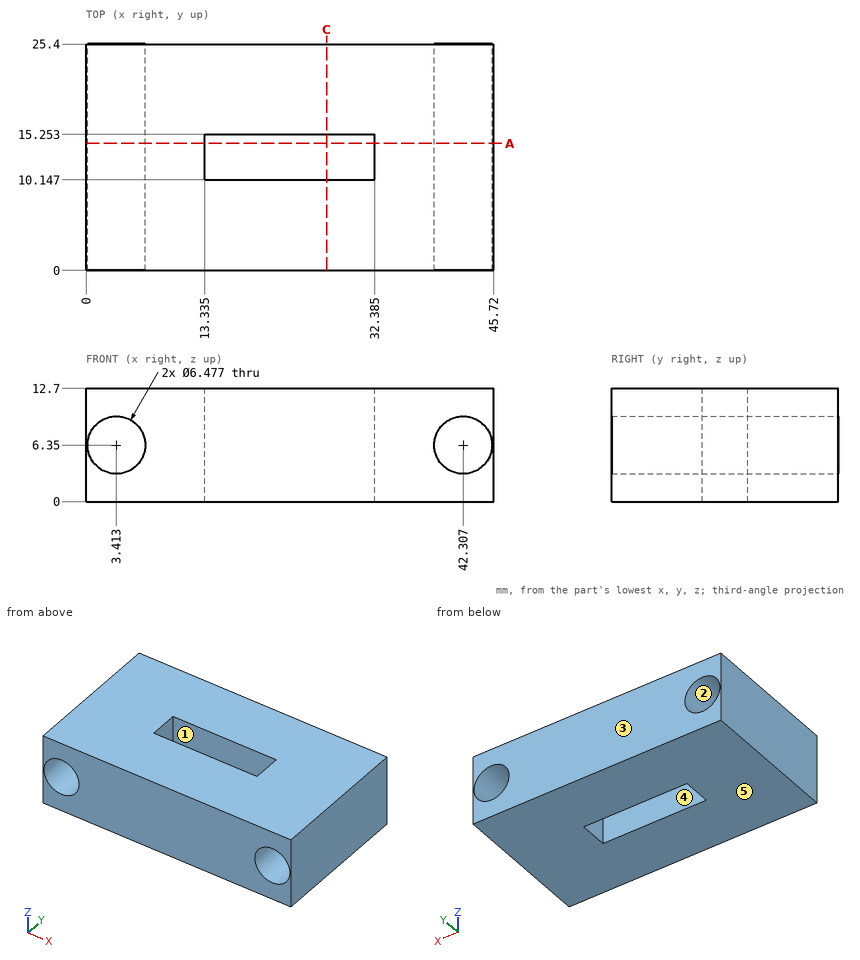
Source: three-view drawing plus pictorial views. Frame: mm from the lowest corner of the part. A direction names the side the tool comes from. Round coordinates to 2 decimals unless told otherwise and drop trailing zeros. Loops run counter-clockwise (first coordinate to the right, second up) from the corner with the lowest first, then second, coordinate; pieces in that order, holes last.
Q1. Section A-A on y = 14.25. State how many separate pieces and enclosed holes the cut face has, plus the area to 3 significant figures.
Q2. Section C-C on x = 27. Return loops of the section in (y, z), plus the area to 3 significant figures.
Q3. Access query for the marked faces 1 and 2. Directions: +Z, -Z, +X, -X, +Y, -Y. A direction counts if a zero-diameter tool reaches every point of the face in a straight line with its end or side. Return the directions, or none.
Q4. Pull-direction query (Y, two-part tool) for the marked faces 3, 4 and 5; classes: released by +Y, released by -Y, zero draft, split by the parting line, or undercut.
Q5. Material intervals for L1, parallel to X at y = 2, z = 6.25; L2, parallel to Y at x = 30.5, z = 7.75; L3, parallel to X at y = 14.5, z = 4 (1 decimal), sorted ascending.
Evaluation:
1. separate pieces: 2
1. enclosed holes: 2
1. area: 273 mm2
2. outline: (0, 0) - (10.15, 0) - (10.15, 12.7) - (0, 12.7) - close; (15.25, 0) - (25.4, 0) - (25.4, 12.7) - (15.25, 12.7) - close
2. area: 258 mm2
3. face 1: +Z, -Z
3. face 2: +Y, -Y
4. face 3: released by +Y
4. face 4: undercut
4. face 5: zero draft
5. L1: x = 0 to 0.18, 6.65 to 39.07, 45.54 to 45.72
5. L2: y = 0 to 10.15, 15.25 to 25.4
5. L3: x = 0 to 1.2, 5.6 to 13.3, 32.4 to 40.1, 44.5 to 45.7
